```python
from build123d import *

# Parameters (mm, degrees)
SKETCH_W        = 61.5
SKETCH_H        = 15
PAD_DEPTH       = 2
SKETCH001_W     = 2
SKETCH001_H     = 15
PAD001_DEPTH    = 59.5
FILLET_R        = 1.5
FILLET001_R     = 1
SKETCH002_R     = 2.2
POCKET_DEPTH    = 2.001
FILLET002_R     = 0.7
SKETCH003_R     = 2.2
POCKET001_DEPTH = 2.001
FILLET003_R     = 0.7


with BuildPart() as part:
    # Sketch → Pad (new body)
    with BuildSketch(Plane.XY):
        Rectangle(SKETCH_W, SKETCH_H)
    extrude(amount=PAD_DEPTH)

    # Sketch001 (on Face6 of Pad) → Pad001 (join)
    with BuildSketch(Plane.XY.offset(2)):
        with Locations((-29.75, 0)):
            Rectangle(SKETCH001_W, SKETCH001_H)
    extrude(amount=PAD001_DEPTH)

    # Fillet
    fillet_edges = [part.edges().sort_by_distance(p)[0] for p in [
        (-30.75, 0, 0),
    ]]
    fillet(fillet_edges, radius=FILLET_R)

    # Fillet001
    fillet001_edges = [part.edges().sort_by_distance(p)[0] for p in [
        (-28.75, 0, 2),
    ]]
    fillet(fillet001_edges, radius=FILLET001_R)

    # Sketch002 (on Face2 of Fillet001) → Pocket (cut, through all)
    with BuildSketch(Plane.XY.offset(2)):
        with Locations((23.05, 0)):
            Circle(SKETCH002_R)
        with Locations((-10.95, 0)):
            Circle(SKETCH002_R)
    extrude(amount=-POCKET_DEPTH, mode=Mode.SUBTRACT)

    # Fillet002
    fillet002_edges = [part.edges().sort_by_distance(p)[0] for p in [
        (20.85, 0, 2),
        (-13.15, 0, 2),
    ]]
    fillet(fillet002_edges, radius=FILLET002_R)

    # Sketch003 (on Face14 of Fillet002) → Pocket001 (cut, through all)
    with BuildSketch(Plane.YZ.offset(-28.75)):
        with Locations((0, 53.8)):
            Circle(SKETCH003_R)
        with Locations((0.10123, 19.8)):
            Circle(SKETCH003_R)
    extrude(amount=-POCKET001_DEPTH, mode=Mode.SUBTRACT)

    # Fillet003
    fillet003_edges = [part.edges().sort_by_distance(p)[0] for p in [
        (-28.75, -2.2, 53.8),
        (-28.75, -2.09877, 19.8),
    ]]
    fillet(fillet003_edges, radius=FILLET003_R)


solid = part.part
```
Can you work these out from the model? Positions are in its coordinate system, mm. A direction names the side the tool comes from. Round coordinates to 2 decimals unless told otherwise and drop trailing zeros. Loops run counter-clockwise (first coordinate to the right, second up) from the corner with the lowest first, then second, coordinate; pieces in that order, holes last. Notation, with made-up numbers: M 83,51 L 106,51 A29 ccw 106,76 Z; hole C 61,33.25 d2. An arc over 180 degrees is marked long. Answer as a JSON object with one key per item and string values. Group by question number.
Q1. On a 3-axis mill with a long thin cutter (end or side, diameter ignored), from which of +Z, -Z, +X, -X, +Y, -Y can I reach the whole of each face in a straight line? I mean faces 1 (the flat face through (30.75, 0, 1)), 2 (the flat face through (-28.75, 0, 32)). Say none if no direction works.
Q2. Imagine slicing it at B-B, the plane z = 19.8. Please give me the cut outline in (x, y).
Q3. Will these pins go through, and if not, where does the flat tip stop? pin 1 (7.5 mm diameter, centred on x = 14.5, y = -3, fed in from +Z); pin 2 (3.5 mm diameter, centred on y = 0.1, z = 19.8, fed in from -X); pin 3 (7.5 mm diameter, centred on y = 2.5, z = 44.5, fed in from +X).
Q4. Imagine slicing it at A-A, the plane x = 23.05. Please give me the cut outline in (y, z), then the cut area to 3 significant figures.
Q5. Imagine slicing it at D-D, the plane y = 0. Count the separate pieces of the cut face and the enclosed holes in it, then the cut area to 3 significant figures.
Q6. Please list where these lines run through material, in increasing order: L1, parallel to Y at x = 23.05, z = 0.75; L2, parallel to Z at x = -18.5, y = -4.5; L3, parallel to X at y = 4, z = 57.
Q7. Imagine slicing it at C-C, the plane y = -4.75. Please give me the cut outline in (x, z), then the cut area to 3 significant figures.
Q8. We'd pull the mould along Z, two halves only. Please class faces 3 (the flat face through (-30, -7.5, 17)), 4 (the flat face through (1, 0, 2)), 5 (the cylindrical face through (-30.09, 1.12, 17.85)): +Z half, -Z half, draft (parallel to the pull), parting line (faces both ways), or undercut.
Findings:
{
 "1": {"face 1": "+Z, -Z, +X, +Y, -Y", "face 2": "+Z, +X, +Y, -Y"},
 "2": {"outline": "M -30.75,-7.5 L -28.75,-7.5 L -28.75,-2.8 A0.7 ccw -29.45,-2.1 L -30.75,-2.1 Z; M -30.75,2.3 L -29.45,2.3 A0.7 ccw -28.75,3 L -28.75,7.5 L -30.75,7.5 Z"},
 "3": {"pin 1": "stops at z = 2", "pin 2": "passes through", "pin 3": "stops at x = -28.75"},
 "4": {"outline": "M -7.5,0 L -2.2,0 L -2.2,1.3 A0.7 ccw -2.9,2 L -7.5,2 Z; M 2.2,0 L 7.5,0 L 7.5,2 L 2.9,2 A0.7 ccw 2.2,1.3 Z", "area": "21.0 mm2"},
 "5": {"separate pieces": "5", "enclosed holes": "0", "area": "206 mm2"},
 "6": {"L1": "y = -7.5 to -2.2, 2.2 to 7.5", "L2": "z = 0 to 2", "L3": "x = -30.75 to -28.75"},
 "7": {"outline": "M -30.75,1.5 A1.5 ccw -29.25,0 L 30.75,0 L 30.75,2 L -27.75,2 A1 cw -28.75,3 L -28.75,61.5 L -30.75,61.5 Z", "area": "242 mm2"},
 "8": {"face 3": "draft", "face 4": "+Z half", "face 5": "undercut"}
}
